For this review, take the finished solid that the model builds, in its own axes (mm). A direction names the side the tool comes from. Round coordinates to 2 decimals unless told otherwise and drop trailing zeros. Order: outer loops, then holes, each group sorted by start corner. A loop starts at its lowest first (then second) coordinate and runs counter-clockwise, first axis right, second up. Notation, with made-up numbers: (21.25, -40) -> (55.25, -40) arc R25 ccw to (55.25, -4) -> close; hole circle Ø5 at (-15.5, -21). An arc over 180 degrees is marked (long way). Answer in a Markdown table with one row per item.
```python
from build123d import *

# Parameters (mm, degrees)
SKETCH_1_R          = 5
EXTRUDE_1_DEPTH     = 25
SKETCH_2_OUTSIDE_W  = 17.744
SKETCH_2_OUTSIDE_H  = 17.744
CUT_EXTRUDE_1_DEPTH = 15
EXTRUDE_START       = 10
SKETCH_3_R          = 5
EXTRUDE_2_DEPTH     = 10


with BuildPart() as part:
    # 스케치1 → 보스-돌출1 (new body)
    with BuildSketch(Plane.XY):
        Circle(SKETCH_1_R)
    extrude(amount=EXTRUDE_1_DEPTH)

    # 스케치2 outside → 컷-돌출1 (cut)
    with BuildSketch(Plane.XY.offset(25)):
        Rectangle(SKETCH_2_OUTSIDE_W, SKETCH_2_OUTSIDE_H)
        with BuildLine():
            Line((-3.5, 3.570714214), (-3.5, -3.570714214))
            ThreePointArc((-3.5, -3.570714214), (5, 0), (-3.5, 3.570714214))
        make_face(mode=Mode.SUBTRACT)
    extrude(amount=-CUT_EXTRUDE_1_DEPTH, mode=Mode.SUBTRACT)

    # 스케치3 → 보스-돌출2 (add)
    with BuildSketch(Plane(origin=(0, 0, 0), x_dir=(-1, 0, 0), z_dir=(0, 0, -1)).offset(EXTRUDE_START)):
        Circle(SKETCH_3_R)
    extrude(amount=-EXTRUDE_2_DEPTH)


solid = part.part
```
Q1. Take a section at A-A, the plane y = 0. Write out the cut boundary in (x, z).
Answer key:
| item | result |
|---|---|
| outline | (-5, -10) -> (5, -10) -> (5, 25) -> (-3.5, 25) -> (-3.5, 10) -> (-5, 10) -> close |
Q2. To check wall thickness, follow probe 1 along X at (y, z) = (-3.5, 11); probe 2 along X at (y, z) = (-3, 17); probe 3 along Y at (x, z) = (-3.75, 2.5). State the ranges of each line that lie inside material, in increasing order.
Answer key:
| item | result |
|---|---|
| probe 1 | x = -3.5 to 3.57 |
| probe 2 | x = -3.5 to 4 |
| probe 3 | y = -3.31 to 3.31 |
Q3. Take a section at D-D, the plane y = -4. Write out the cut boundary in (x, z), then the cut area to 3 significant figures.
Answer key:
| item | result |
|---|---|
| outline | (-3, -10) -> (3, -10) -> (3, 25) -> (-3, 25) -> close |
| area | 210 mm^2 |
Q4. Clearance check with flat-ended pins moving along their axes: pin 1 Ø0.8 at (x, y) = (-4, 1) entering from +Z; pin 2 Ø3 at (y, z) = (-0.5, 9) entering from -X; pin 3 Ø3.5 at (y, z) = (-0.5, 19.5) entering from -X; pin 4 Ø1 at (y, z) = (3.5, 5) entering from -X. State where each tip first meets the part, or that it passes through.
Answer key:
| item | result |
|---|---|
| pin 1 | stops at z = 10 |
| pin 2 | stops at x = -5 |
| pin 3 | stops at x = -3.5 |
| pin 4 | stops at x = -4 |
Q5. Tool access review of faces 1 (the face through (1, 0, 25)), 2 (the face through (-4, 0, 10)): name each direction out of +Z, -Z, +X, -X, +Y, -Y from which nothing blocks a thin tool from reaching the whole face with its end or side.
Answer key:
| item | result |
|---|---|
| face 1 | +Z, +X, -X, +Y, -Y |
| face 2 | +Z, -X, +Y, -Y |
Q6. Take a section at B-B, the plane z = 1. Write out the cut boundary in (x, y).
Answer key:
| item | result |
|---|---|
| outline | circle Ø10 at (0, 0) |
Q7. Take a section at C-C, the plane x = -4.5. Write out the cut boundary in (y, z).
Answer key:
| item | result |
|---|---|
| outline | (-2.18, -10) -> (2.18, -10) -> (2.18, 10) -> (-2.18, 10) -> close |
